Autodesk Inventor part; units mm, degrees
ref_plane "YZ Plane" through (0, 0, 0) normal (1, 0, 0) x (0, 1, 0)
ref_plane "XZ Plane" through (0, 0, 0) normal (0, 1, 0) x (-1, 0, 0)
ref_plane "XY Plane" through (0, 0, 0) normal (0, 0, 1) x (1, 0, 0)
sketch "草图1" plane through (0, 0, 0) normal (0, 0, 1) x (1, 0, 0)
  circle A0 centre (0, 0) radius 5
  circle A1 centre (260, 0) radius 5
  line L0 (-10, 15) -> (10, 15)
  line L1 (10, 15) -> (10, -15)
  line L2 (10, -15) -> (-10, -15)
  line L3 (-10, -15) -> (-10, 15)
  line L4 (250, 15) -> (270, 15)
  line L5 (270, 15) -> (270, -15)
  line L6 (270, -15) -> (250, -15)
  line L7 (250, -15) -> (250, 15)
  line L8 (-30, 25) -> (290, 25)
  line L9 (290, 25) -> (290, 15)
  line L10 (290, 15) -> (-30, 15)
  line L11 (-30, 15) -> (-30, 25)
  dimension "d0" = 10
  dimension "d1" = 10
  dimension "d2" = 260
  dimension "d3" = 20
  dimension "d4" = 10
  dimension "d5" = 30
  dimension "d6" = 15
  dimension "d7" = 20
  dimension "d8" = 30
  dimension "d9" = 15
  dimension "d10" = 10
  dimension "d11" = 320
  dimension "d12" = 20
  dimension "d13" = 10
extrude "拉伸1" add sketch "草图1" along normal blind 30 contours A1 | L0 L1 L2 L3 | L4 L5 L6 L7
extrude "拉伸2" add sketch "草图1" along normal blind 145 and the other way blind 115 contours L10 L11 L8 L9 L4 L0
extrude "拉伸3" cut sketch "草图1" along normal blind 30 contours A1
sketch "草图2" plane through (-30, 15, 145) normal (0, -1, 0) x (1, 0, 0)
  line L0 (309.6956, -155) -> (317.1956, -155)
  line L1 (317.1956, -155) -> (317.1956, -105)
  line L2 (317.1956, -105) -> (309.6956, -105)
  line L3 (309.6956, -105) -> (309.6956, -155)
  line L4 (0, 0) -> (320, 0)
  point P0 (30, -145)
  dimension "d22" = 7.5
  dimension "d23" = 105
  dimension "d24" = 50
extrude "拉伸4" add sketch "草图2" along normal blind 7
sketch "草图3" plane through (287.1956, 15, 40) normal (1, 0, 0) x (0, 0, -1)
  line L0 (50, 0) -> (50, -7)
  line L1 (0, 0) -> (0, -7)
  line L2 (50, -7) -> (0, -7)
  line L3 (0, -7) -> (0, -5)
  line L4 (0, -5) -> (50, -5)
  line L5 (50, -5) -> (50, -7)
  point P0 (40, -15)
  dimension "d27" = 2
extrude "拉伸5" add sketch "草图3" along normal blind 12
properties part number "滑台"
Read the model definition and answer for the solid it produces. Units are mm, in the model's axes. A direction names the side the tool comes from. Coordinates: 2 decimals unless noted, no trailing zeros. Write each loop counter-clockwise with the first axis right and the second up, starting at its lowest first coordinate (ties: lowest second). Pieces come first, ordered by that corner, then holes. Notation, with made-up numbers: (55.25, -14) - (109.25, -14) arc R15 cw to (109.25, -3) - close; hole circle Ø3 at (49, 80). An arc over 180 degrees is marked (long way). Answer as a JSON object with one key per item and string values. Group by question number.
1. A cutting plane is placed at D-D (x = 62.5). Determine the outline of the cut face in (y, z).
2. A cutting plane is placed at C-C (z = -20). Determine the outline of the cut face in (x, y), plus the area to 3 significant figures.
3. Each of these flat-tipped pins is pushed along its axis until it touches: P1, Ø9, axis at y = -3.5, z = 21, coming from the -X side; P2, Ø13, axis at x = 260, y = 0, coming from the -Z side; P3, Ø8, axis at y = 21.5, z = 71, coming from the +X side. Where does it stop, or does it pass through?
4. The mould has two halves that part along X. Classify faces 1 (the flat face through (-10, 0, 15)), 2 (the flat face through (287, 11, 40)), 3 (the flat face through (10, 0, 15)): +X half, -X half, draft (parallel to the pull), parting line (faces both ways), or undercut.
5. A cutting plane is placed at B-B (x = 0). Determine the outline of the cut face in (y, z).
6. Consider L1, parallel to Y at x = 0, z = 15; L2, parallel to Y at x = 278.5, z = -76.5; L3, parallel to X at y = -13, z = 1.5. Determine where each line is inside the solid, lowest interval first. Write a range as [from, to].
7. A cutting plane is placed at A-A (y = -10). Determine the outline of the cut face in (x, z), plus the area to 3 significant figures.
8. Which of the six approach directions +Z, -Z, +X, -X, +Y, -Y give full straight-line access (tool end or side, diameter ignored) to faces 4 (the flat face through (293, 10, 15)), 5 (the flat face through (279.696, 12, 15)), 6 (the flat face through (4, 4, 30))?
Worked out:
{
 "1": {"outline": "(15, -115) - (25, -115) - (25, 145) - (15, 145) - close"},
 "2": {"outline": "(-30, 15) - (290, 15) - (290, 25) - (-30, 25) - close", "area": "3,200 mm²"},
 "3": {"P1": "stops at x = -10", "P2": "stops at z = 0", "P3": "stops at x = 290"},
 "4": {"face 1": "-X half", "face 2": "draft", "face 3": "undercut"},
 "5": {"outline": "(-15, 0) - (-5, 0) - (-5, 30) - (-15, 30) - close; (5, 0) - (15, 0) - (15, -115) - (25, -115) - (25, 145) - (15, 145) - (15, 30) - (5, 30) - close"},
 "6": {"L1": "y = [-15, -5], [5, 25]", "L2": "y = [15, 25]", "L3": "x = [-10, 10], [250, 270]"},
 "7": {"outline": "(-10, 0) - (10, 0) - (10, 30) - (-10, 30) - close; (250, 0) - (270, 0) - (270, 30) - (250, 30) - close", "area": "1,200 mm²"},
 "8": {"face 4": "+Z, -Z, +X", "face 5": "+Z, -Z, -Y", "face 6": "+Z, -X, -Y"}
}
